Here's the drawing with two shaded views (mm, measured from the low corner). I have some questions. Coordinates: 2 decimals unless noted, no trailing zeros. Write each loop counter-clockwise with the first axis right and the second up, starting at its lowest first coordinate (ties: lowest second). Pieces come first, ordered by that corner, then holes.
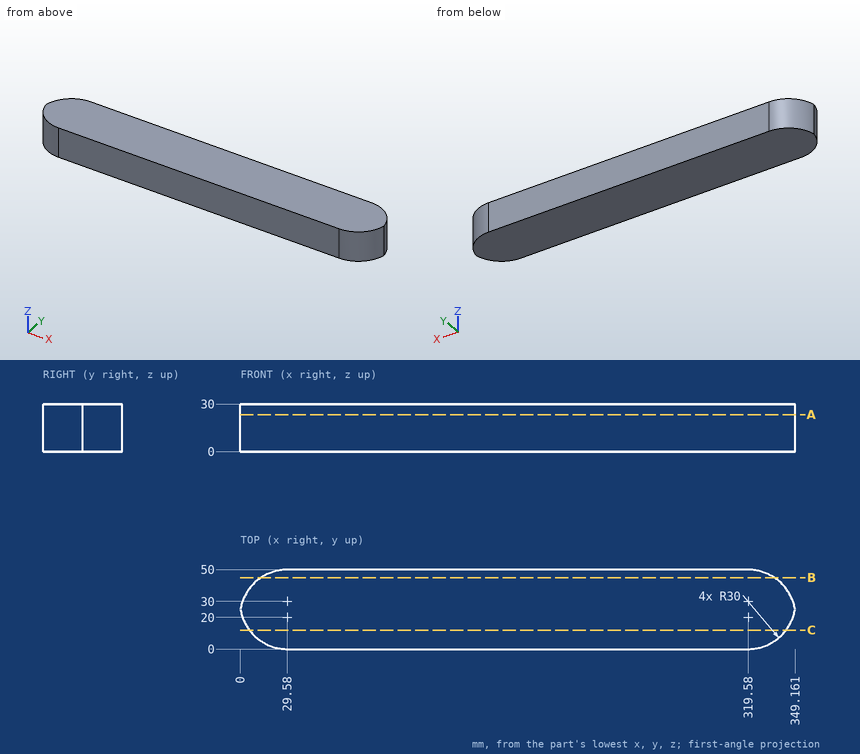
1. I want a section at C-C on y = 12. Please give me the cut outline in (x, z).
Verdict:
outline: (5.58, 0) - (343.58, 0) - (343.58, 30) - (5.58, 30) - close
2. I want a section at B-B on y = 45. Please give me the cut outline in (x, z).
Verdict:
outline: (13, 0) - (336.16, 0) - (336.16, 30) - (13, 30) - close
3. Please list where these lines run through material, in increasing order: line 1 along X through (y, z) = (10.5, 28); line 2 along X through (y, z) = (40.5, 21.75) (1 decimal); line 3 along Y through (x, z) = (324.5, 14.5).
Verdict:
line 1: x = 6.78 to 342.38
line 2: x = 7.7 to 341.5
line 3: y = 0.41 to 49.59
4. For pin 1 (6 mm diameter, centred on y = 17.5, z = 21, fed in from -X) (1 decimal); pin 2 (3 mm diameter, centred on y = 40, z = 14.5, fed in from -X) (1 decimal); pin 3 (3 mm diameter, centred on y = 5, z = 8, fed in from -X), each with a flat end and sliding along its axis, tell me the tip position at first contact or that it passes through.
Verdict:
pin 1: stops at x = 1.1
pin 2: stops at x = 6
pin 3: stops at x = 10.93
5. I want a section at A-A on z = 23.25. Please give me the cut outline in (x, y), plus the area to 3 significant figures.
Verdict:
outline: (0, 25) arc R30 ccw to (29.58, 0) - (319.58, 0) arc R30 ccw to (349.16, 25) arc R30 ccw to (319.58, 50) - (29.58, 50) arc R30 ccw to start
area: 16,700 mm2
